Input: part model. Units: mm. Frame: model coordinates. Face numbers are marked on the shaded views. A direction names the side the tool comes from. Coordinates: 2 decimals unless noted, no trailing zeros. Write each loop counter-clockwise with the first axis right and the second up, starting at its lowest first coordinate (ties: lowest second). Pieces come first, ordered by that corner, then holes. Notation, with made-up numbers: (11, 7.5) - (54, 7.5) arc R16 ccw to (54, 31.5) - close; hole circle Ø8 at (61.5, 76). An arc over 180 degrees is marked (long way). One line per question, with ' | ' between items. Start each with the question number.
1) Section query C-C on z = -3. Return loops of the section in (x, y) (1 decimal).
2) Section query D-D on y = 4.5. Give the number of separate pieces and of enclosed holes in the cut face, and give its area (3 significant figures).
3) Section query A-A on y = 0. Return loops of the section in (x, z).
4) First-contact query: P1, Ø1.5, axis at x = 4, y = -3.5, coming from the -Z side; P2, Ø7, axis at x = 0, y = 0, coming from the -Z side; P3, Ø1.5, axis at y = 8.5, z = 3, coming from the -X side; P4, Ø4, axis at x = 1, y = 2, coming from the -Z side. Flat tips, straight axial feed; report the tip coordinate or a pass-through.
5) Line query: line 1 (X direction, y = 4.75, z = 4.25); line 2 (Y direction, x = -5.25, z = -1.75); line 3 (X direction, y = -4.25, z = -3.25). Output: solid intervals per line, ascending.
6) Reachability of the marked faces 4, 5 and 6 from +Z, -Z, +X, -X, +Y, -Y: full face, straight path, thin tool, end or side. Return the list, or none.
7) Draft query along Z for the marked faces 1, 2 and 3. Return one class per face: released by +Z, released by -Z, zero draft, split by the parting line, or undercut.
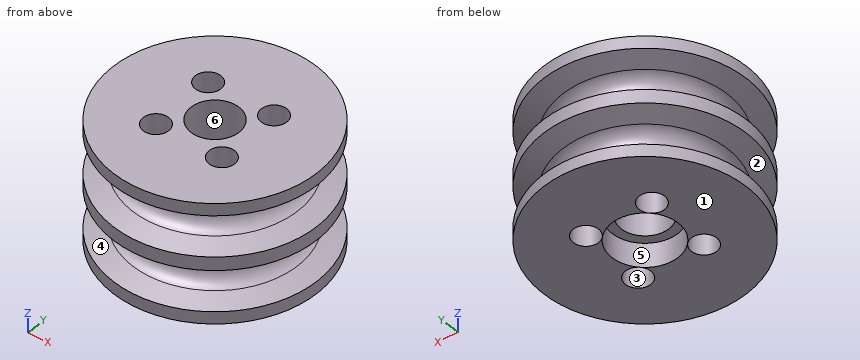
```python
from build123d import *

# Parameters (mm, degrees)
SKETCH2_R          = 1.5875
CUT_EXTRUDE1_DEPTH = 14.984431


with BuildPart() as part:
    # Sketch1 → Revolve1 (revolve)
    with BuildSketch(Plane(origin=(0, 0, 0), x_dir=(0, 0, -1), z_dir=(1, 0, 0))):
        with BuildLine():
            Line((-1.488284524, 10.287553907), (-0.841871541, 12.7))
            Line((-0.841871541, 12.7), (0.841871541, 12.7))
            Line((0.841871541, 12.7), (1.488284524, 10.287553907))
            ThreePointArc((1.488284524, 10.287553907), (3.405043585, 8.81677295), (5.321802647, 10.287553907))
            Line((5.321802647, 10.287553907), (5.968215629, 12.7))
            Line((5.968215629, 12.7), (7.492215629, 12.7))
            Line((7.492215629, 12.7), (7.492215629, 4.127000001))
            Line((7.492215629, 4.127000001), (4.492215629, 4.127000001))
            Line((4.492215629, 4.127000001), (4.492215629, 3))
            Line((4.492215629, 3), (-7.492215629, 3))
            Line((-7.492215629, 3), (-7.492215629, 12.7))
            Line((-7.492215629, 12.7), (-5.968215629, 12.7))
            Line((-5.968215629, 12.7), (-5.321802647, 10.287553907))
            ThreePointArc((-5.321802647, 10.287553907), (-3.405043585, 8.81677295), (-1.488284524, 10.287553907))
        make_face()
    revolve(axis=Axis((0, 0, 0), (0, 0, -1)))

    # Sketch2 → Cut-Extrude1 (cut)
    with BuildSketch(Plane(origin=(0, 0, -7.492215629), x_dir=(-1, 0, 0), z_dir=(0, 0, -1))):
        with Locations((4.041115254, 4.041115254)):
            Circle(SKETCH2_R)
        with Locations((-4.041115254, 4.041115254)):
            Circle(SKETCH2_R)
        with Locations((-4.041115254, -4.041115254)):
            Circle(SKETCH2_R)
        with Locations((4.041115254, -4.041115254)):
            Circle(SKETCH2_R)
    extrude(amount=-CUT_EXTRUDE1_DEPTH, mode=Mode.SUBTRACT)


solid = part.part
```
Answer key:
1) outline: circle Ø17.7 at (0, 0); hole circle Ø3.2 at (-4, -4); hole circle Ø3.2 at (-4, 4); hole circle Ø6 at (0, 0); hole circle Ø3.2 at (4, -4); hole circle Ø3.2 at (4, 4)
2) separate pieces: 3 | enclosed holes: 0 | area: 199 mm²
3) outline: (-12.7, -7.49) - (-4.13, -7.49) - (-4.13, -4.49) - (-3, -4.49) - (-3, 7.49) - (-12.7, 7.49) - (-12.7, 5.97) - (-10.29, 5.32) arc R1.98 cw to (-10.29, 1.49) - (-12.7, 0.84) - (-12.7, -0.84) - (-10.29, -1.49) arc R1.98 cw to (-10.29, -5.32) - (-12.7, -5.97) - close; (3, -4.49) - (4.13, -4.49) - (4.13, -7.49) - (12.7, -7.49) - (12.7, -5.97) - (10.29, -5.32) arc R1.98 cw to (10.29, -1.49) - (12.7, -0.84) - (12.7, 0.84) - (10.29, 1.49) arc R1.98 cw to (10.29, 5.32) - (12.7, 5.97) - (12.7, 7.49) - (3, 7.49) - close
4) P1: through | P2: z = -4.49 | P3: x = -4.36 | P4: z = -7.49
5) line 1: -7.65 to -5.46, -2.62 to 2.62, 5.46 to 7.65 | line 2: -8.16 to -5.07, -3.01 to 3.01, 5.07 to 8.16 | line 3: -7.73 to -5.61, -2.47 to 2.47, 5.61 to 7.73
6) face 4: none | face 5: -Z | face 6: +Z, -Z
7) face 1: released by -Z | face 2: undercut | face 3: zero draft
